from build123d import *

# Parameters (mm, degrees)
CROQUIS1_R              = 32
SALIENTE_EXTRUIR1_DEPTH = 5
SALIENTE_EXTRUIR2_DEPTH = 2
CROQUIS3_R              = 1.7
CORTAR_EXTRUIR1_DEPTH   = 19
CROQUIS4_R              = 2.95
CORTAR_EXTRUIR2_DEPTH   = 3
CROQUIS5_R              = 1.7
CORTAR_EXTRUIR3_DEPTH   = 5
CROQUIS9_R              = 75
CORTAR_EXTRUIR6_DEPTH   = 37


with BuildPart() as part:
    # Croquis1 → Saliente-Extruir1 (new body)
    with BuildSketch(Plane(origin=(0, 0, 0), x_dir=(1, 0, 0), z_dir=(0, 1, 0))):
        with BuildLine():
            ThreePointArc((-47.29361892, 36.923076923), (0, -60), (47.29361892, 36.923076923))
            ThreePointArc((47.29361892, 36.923076923), (32.46950766, 80), (47.29361892, 123.076923077))
            ThreePointArc((47.29361892, 123.076923077), (0, 220), (-47.29361892, 123.076923077))
            ThreePointArc((-47.29361892, 123.076923077), (-32.46950766, 80), (-47.29361892, 36.923076923))
        make_face()
        Circle(CROQUIS1_R, mode=Mode.SUBTRACT)
        with Locations((0, 160)):
            Circle(CROQUIS1_R, mode=Mode.SUBTRACT)
    extrude(amount=SALIENTE_EXTRUIR1_DEPTH)

    # Croquis2 → Saliente-Extruir2 (add)
    with BuildSketch(Plane(origin=(0, 5, 0), x_dir=(1, 0, 0), z_dir=(0, 1, 0))):
        with BuildLine():
            Line((5, 205), (-5, 205))
            Line((-5, 205), (-5, 219.791303716))
            ThreePointArc((-5, 219.791303716), (0, 220), (5, 219.791303716))
            Line((5, 219.791303716), (5, 205))
        make_face()
        with BuildLine():
            Line((-5, -45), (5, -45))
            Line((5, -45), (5, -59.791303716))
            ThreePointArc((5, -59.791303716), (0, -60), (-5, -59.791303716))
            Line((-5, -59.791303716), (-5, -45))
        make_face()
    extrude(amount=SALIENTE_EXTRUIR2_DEPTH)

    # Croquis3 → Cortar-Extruir1 (cut)
    with BuildSketch(Plane(origin=(0, 7, 0), x_dir=(1, 0, 0), z_dir=(0, 1, 0))):
        with Locations((0, 215)):
            Circle(CROQUIS3_R)
        with Locations((0, -55)):
            Circle(CROQUIS3_R)
    extrude(amount=-CORTAR_EXTRUIR1_DEPTH, mode=Mode.SUBTRACT)

    # Croquis4 → Cortar-Extruir2 (cut)
    with BuildSketch(Plane.XZ):
        with Locations((0, 55)):
            Circle(CROQUIS4_R)
        with Locations((0, -215)):
            Circle(CROQUIS4_R)
    extrude(amount=-CORTAR_EXTRUIR2_DEPTH, mode=Mode.SUBTRACT)

    # Croquis5 → Cortar-Extruir3 (cut)
    with BuildSketch(Plane.XZ):
        with Locations((-28.5, -73.5)):
            Circle(CROQUIS5_R)
        with Locations((-28.5, -86.5)):
            Circle(CROQUIS5_R)
        with Locations((28.5, -86.5)):
            Circle(CROQUIS5_R)
        with Locations((28.5, -73.5)):
            Circle(CROQUIS5_R)
    extrude(amount=-CORTAR_EXTRUIR3_DEPTH, mode=Mode.SUBTRACT)

    # Croquis9 → Cortar-Extruir6 (cut)
    with BuildSketch(Plane.XZ):
        with Locations((0, -160)):
            Circle(CROQUIS9_R)
    extrude(amount=-CORTAR_EXTRUIR6_DEPTH, mode=Mode.SUBTRACT)


solid = part.part
The model under review builds one solid part; all positions refer to its coordinate system, in mm. A direction names the side the tool comes from. Round coordinates to 2 decimals unless told otherwise and drop trailing zeros. Write each loop counter-clockwise with the first axis right and the second up, starting at its lowest first coordinate (ties: lowest second). Pieces come first, ordered by that corner, then holes. Notation, with made-up numbers: M -34.75,-26.5 L -17.75,-26.5 A13 cw -17.75,-14.5 Z; hole C 53.5,-20.75 d10. An arc over 180 degrees is marked long. Use a Markdown table: item, result. Add a question column.
Q1. We need section B-B, the plane y = 1.25. State the section outline as (x, z) points, plus the area to 3 significant figures.
Q2. We need section C-C, the plane z = 0. State the section outline as (x, y) points.
Q3. We need section D-D, the plane z = -73.5. State the section outline as (x, y) points, plus the area to 3 significant figures.
Q4. Insertion check: pin 1 (5.5 mm diameter, centred on x = 28.5, z = -86.5, fed in from -Y); pin 2 (1 mm diameter, centred on x = 2.5, y = 6.5, fed in from -Z); pin 3 (0.6 mm diameter, centred on y = 6, z = 51, fed in from -X); pin 4 (0.6 mm diameter, centred on y = 6.5, z = 54, fed in from +X). Each pin has a flat end and moves straight along its axis. Give the tip position at first contact, or say it passes through.
Q5. Machinability: for faces 1 (the face through (0, 3, 53)), 2 (the face through (30.07, 2.46, -74.15)), which of the approach directions +Z, -Z, +X, -X, +Y, -Y give a long, thin tool a straight path to every point of the face, cutting with its end or side? Answer none if there is none.
Q6. We need section A-A, the plane x = 0. State the section outline as (y, z) points, plus the area to 3 significant figures.
Q7. To check wall thickness, follow line 1 (Z direction, x = 0, y = 3.25); line 2 (Z direction, x = 0.5, y = 3.25); line 3 (Z direction, x = 28.5, y = 1.25). State the ranges of each line that lie inside material, in increasing order.
Q8. The part is to be moulded in two halves that separate along X. For faces 3 (the face through (-34.35, 2.46, -63.89)), 4 (the face through (34.544, 2.465, -63.085)), 5 (the face through (-1.25, 5.03, 53.85)), 6 (the face through (-1, 0, -35)), say which applies: pulls with the +X half, pulls with the -X half, needs draft (parallel to the pull), parting line crosses it, or undercut.
Findings below:
| question | item | result |
|---|---|---|
| 1 | outline | M -47.29,-36.92 A70 cw -33.69,-92.99 A75 cw 33.69,-92.99 A70 cw 47.29,-36.92 A60 ccw long Z; hole C 0,0 d64; hole C -28.5,-86.5 d3.4; hole C -28.5,-73.5 d3.4; hole C 0,55 d5.9; hole C 28.5,-86.5 d3.4; hole C 28.5,-73.5 d3.4 |
| 1 | area | 10,200 mm² |
| 2 | outline | M -60,0 L -32,0 L -32,5 L -60,5 Z; M 32,0 L 60,0 L 60,5 L 32,5 Z |
| 3 | outline | M -32.77,0 L -30.2,0 L -30.2,5 L -32.77,5 Z; M -26.8,0 L 26.8,0 L 26.8,5 L -26.8,5 Z; M 30.2,0 L 32.77,0 L 32.77,5 L 30.2,5 Z |
| 3 | area | 294 mm² |
| 4 | pin 1 | stops at y = 0 |
| 4 | pin 2 | stops at z = 45 |
| 4 | pin 3 | stops at x = -5 |
| 4 | pin 4 | stops at x = 5 |
| 5 | face 1 | -Y |
| 5 | face 2 | +Y, -Y |
| 6 | outline | M 0,-85 L 5,-85 L 5,-32 L 0,-32 Z; M 0,32 L 5,32 L 5,45 L 7,45 L 7,53.3 L 3,53.3 L 3,52.05 L 0,52.05 Z; M 0,57.95 L 3,57.95 L 3,56.7 L 7,56.7 L 7,60 L 0,60 Z |
| 6 | area | 404 mm² |
| 7 | line 1 | z = -85 to -32, 32 to 53.3, 56.7 to 60 |
| 7 | line 2 | z = -85 to -32, 32 to 53.38, 56.62 to 60 |
| 7 | line 3 | z = -90.63 to -88.2, -84.8 to -75.2, -71.8 to -14.55, 14.55 to 52.8 |
| 8 | face 3 | pulls with the -X half |
| 8 | face 4 | pulls with the +X half |
| 8 | face 5 | undercut |
| 8 | face 6 | needs draft |
